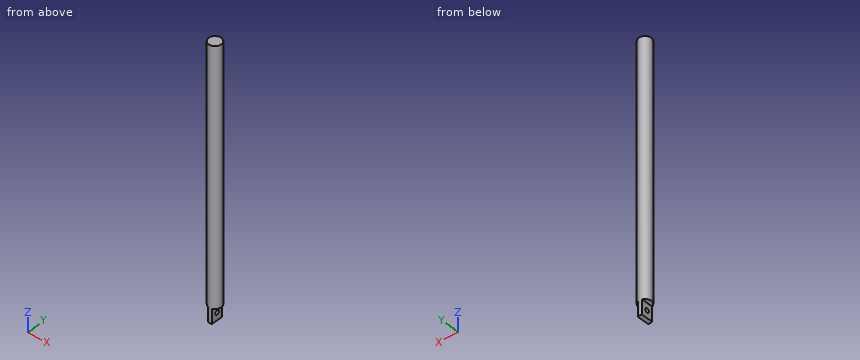
from build123d import *

# Parameters (mm, degrees)
F0_R     = 3
F1_DEPTH = 128
F2_W     = 2
F2_H     = 7
F3_DEPTH = 12.5
F4_R     = 1
F5_DEPTH = 50


with BuildPart() as f1:
    # F0 (on Top) → F1 (new body)
    with BuildSketch(Plane.XY):
        Circle(F0_R)
    extrude(amount=F1_DEPTH)

    # F2 (on Front) → F3 (cut, symmetric)
    with BuildSketch(Plane.XZ):
        with Locations((-2, 3.5)):
            Rectangle(F2_W, F2_H)
        with Locations((2, 3.5)):
            Rectangle(F2_W, F2_H)
    extrude(amount=F3_DEPTH, both=True, mode=Mode.SUBTRACT)

    # F4 (on Right) → F5 (cut, symmetric)
    with BuildSketch(Plane.YZ):
        with Locations((0, 3.561988)):
            Circle(F4_R)
    extrude(amount=F5_DEPTH, both=True, mode=Mode.SUBTRACT)


solid = f1.part
Check sheet for the modelled part. Datum: model origin and axes. Units: mm. Round coordinates to 2 decimals unless told otherwise and drop trailing zeros. Loops run counter-clockwise (first coordinate to the right, second up) from the corner with the lowest first, then second, coordinate; pieces in that order, holes last. Notation, with made-up numbers: M 8.25,25 L 14.25,25 A18 cw 14.25,32 Z; hole C -32,6.25 d3. An arc over 180 degrees is marked long. One line per question, with ' | ' between items. Start each with the question number.
Item 1: Section check B-B (z = 110). Record the boundary of the cut face in (x, y), and give its area (3 significant figures).
Item 2: Scan lines: probe 1 along Z at (x, y) = (-0.3, 0); probe 2 along X at (y, z) = (-0.2, 60); probe 3 along Z at (x, y) = (1.9, 1.05). Record each from-to range of solid material in increasing order.
Item 3: Gauge pin test, flat end, axial feed: pin 1 Ø1 at (x, y) = (-2, -1) entering from -Z. Record the tip position at first contact, or that the pin passes through.
Item 4: Section check A-A (y = 0). Record the boundary of the cut face in (x, z).
Worked out:
1) outline: C 0,0 d6 | area: 28.3 mm^2
2) probe 1: 0 to 2.56, 4.56 to 128 | probe 2: -2.99 to 2.99 | probe 3: 7 to 128
3) pin 1: z = 7
4) outline: M -3,7 L -1,7 L -1,4.56 L 1,4.56 L 1,7 L 3,7 L 3,128 L -3,128 Z; M -1,0 L 1,0 L 1,2.56 L -1,2.56 Z
